For this review, take the finished solid that the model builds, in its own axes (mm). A direction names the side the tool comes from. Give positions to 0.01 mm unless a question says otherwise; leave off trailing zeros. Loops run counter-clockwise (first coordinate to the right, second up) from the corner with the lowest first, then second, coordinate; pieces in that order, holes last. Notation, with made-up numbers: (-27.5, 35.25) - (-22.5, 35.25) arc R36 ccw to (-22.5, 69.25) - close; hole circle Ø7 at (-38.5, 59.25). An arc over 180 degrees is marked (long way). Put each result on its own line as item: value. Start each with the question number.
from build123d import *

# Parameters (mm, degrees)
SKETCH1_W               = 58.6
SKETCH1_H               = 6.25
BOSS_EXTRUDE1_DEPTH     = 30
CUT_EXTRUDE1_DEPTH      = 67.128832592
CUT_EXTRUDE1_DEPTH_BACK = 35
SKETCH4_R               = 2.5
SKETCH4_W               = 15.6
SKETCH4_H               = 10.5
CUT_EXTRUDE2_DEPTH      = 4
CUT_EXTRUDE3_DEPTH      = 9.5
SKETCH6_W               = 15.6
SKETCH6_H               = 1
SKETCH6_H_2             = 0.5
CUT_EXTRUDE4_DEPTH      = 4
FILLET1_R               = 3
SKETCH7_R               = 1.65
CUT_EXTRUDE5_DEPTH      = 3


with BuildPart() as part:
    # Sketch1 → Boss-Extrude1 (new body)
    with BuildSketch(Plane(origin=(0, 0, 0), x_dir=(0, 0, -1), z_dir=(1, 0, 0))):
        with Locations((29.3, 3.125)):
            Rectangle(SKETCH1_W, SKETCH1_H)
    extrude(amount=BOSS_EXTRUDE1_DEPTH)

    # Sketch2 → Cut-Extrude1 (cut, two sides: drawn at the far end of the back side and taken through both)
    with BuildSketch(Plane.XY.offset(-CUT_EXTRUDE1_DEPTH_BACK)):
        with BuildLine():
            Line((5, 6.25), (25, 6.25))
            ThreePointArc((25, 6.25), (15, 2), (5, 6.25))
        make_face()
    extrude(amount=CUT_EXTRUDE1_DEPTH + CUT_EXTRUDE1_DEPTH_BACK, mode=Mode.SUBTRACT)

    # Sketch4 → Cut-Extrude2 (cut)
    with BuildSketch(Plane.XZ):
        with Locations(Location((15, -8.37, 0), (0, 0, 270))):
            Circle(SKETCH4_R)
        with Locations(Location((15, -15.02, 0), (0, 0, 270))):
            Circle(SKETCH4_R)
        with Locations(Location((15, -22.65, 0), (0, 0, 270))):
            Circle(SKETCH4_R)
        with Locations((15, -43.35)):
            Rectangle(SKETCH4_W, SKETCH4_H)
    extrude(amount=-CUT_EXTRUDE2_DEPTH, mode=Mode.SUBTRACT)

    # Sketch5 → Cut-Extrude3 (cut)
    with BuildSketch(Plane(origin=(0, 0, -58.6), x_dir=(-1, 0, 0), z_dir=(0, 0, -1))):
        Polygon((-9.85, 0.95), (-20.15, 0.95), (-17.975, 3.125), (-20.15, 5.3), (-9.85, 5.3), align=None)
    extrude(amount=-CUT_EXTRUDE3_DEPTH, mode=Mode.SUBTRACT)

    # Sketch6 → Cut-Extrude4 (cut)
    with BuildSketch(Plane.XZ):
        with Locations((15, -37.6)):
            Rectangle(SKETCH6_W, SKETCH6_H)
        with Locations((15, -48.85)):
            Rectangle(SKETCH6_W, SKETCH6_H_2)
    extrude(amount=-CUT_EXTRUDE4_DEPTH, mode=Mode.SUBTRACT)

    # Fillet1
    fillet1_edges = [part.edges().sort_by_distance(p)[0] for p in [
        (30, 3.125, -58.6),
        (30, 3.125, 0),
        (0, 3.125, -58.6),
        (0, 3.125, 0),
    ]]
    fillet(fillet1_edges, radius=FILLET1_R)

    # Sketch7 → Cut-Extrude5 (cut)
    with BuildSketch(Plane.XZ):
        with Locations(Location((3, -55.6, 0), (0, 0, 270))):
            Circle(SKETCH7_R)
        with Locations(Location((27, -55.6, 0), (0, 0, 90))):
            Circle(SKETCH7_R)
        with Locations(Location((27, -3, 0), (0, 0, 270))):
            Circle(SKETCH7_R)
        with Locations(Location((3, -3, 0), (0, 0, 90))):
            Circle(SKETCH7_R)
    extrude(amount=-CUT_EXTRUDE5_DEPTH, mode=Mode.SUBTRACT)


solid = part.part
1) Machinability: for faces 1 (the flat face through (0, 3, -29)), 2 (the flat face through (15, 2, -37.1)), 3 (the flat face through (15, 5, -35)), which of the approach directions +Z, -Z, +X, -X, +Y, -Y give a long, thin tool a straight path to every point of the face, cutting with its end or side? Answer none if there is none.
2) Take a section at B-B on z = -30.5. State the section outline as (x, y) points, and give its area (3 significant figures).
3) Wall thickness on probe 1 along Z at (x, y) = (15, 0.65); probe 2 along Z at (x, y) = (18, 0.75); probe 3 along X at (y, z) = (0.85, -15.02): over which ranges is each line inside the solid? List them lowest first.
4) Take a section at C-C on x = 8.75. State the section outline as (y, z) points, and give its area (3 significant figures).
5) Take a section at A-A on z = -22.65. State the section outline as (x, y) points, and give its area (3 significant figures).
6) Mouldability with a two-part tool opening along Y and no side actions: class faces 4 (the cylindrical face through (3.07, 1.48, -53.95)), 5 (the flat face through (27, 3, -56)), 6 (the flat face through (19.05, 4.2, -53.92)), 7 (the flat face through (15, 5.3, -54)) as released by +Y, released by -Y, zero draft, split by the parting line, or undercut.
7) Insertion check: P1, Ø2.5, axis at x = 3, z = -55.6, coming from the -Y side; P2, Ø8, axis at x = 15, z = -22.65, coming from the +Y side; P3, Ø3, axis at x = 15, z = -15.02, coming from the +Y side; P4, Ø6, axis at x = 19, z = -10, coming from the +Y side. Each pin has a flat end and moves straight along its axis. Give the tip position at first contact, or say it passes through.
Answers follow:
1. face 1: +Z, -Z, -X, +Y, -Y
1. face 2: -Y
1. face 3: +Z, +Y
2. outline: (0, 0) - (30, 0) - (30, 6.25) - (25, 6.25) arc R13.89 cw to (5, 6.25) - (0, 6.25) - close
2. area: 129 mm2
3. probe 1: -58.6 to -49.1, -37.1 to -25.15, -20.15 to -17.52, -12.52 to -10.87, -5.87 to 0
3. probe 2: -58.6 to -49.1, -37.1 to 0
3. probe 3: 0 to 12.5, 17.5 to 30
4. outline: (0, -58.6) - (6.25, -58.6) - (6.25, -35) - (3.49, -35) - (3.49, 0) - (0, 0) - (0, -37.1) - (4, -37.1) - (4, -49.1) - (0, -49.1) - close
4. area: 221 mm2
5. outline: (0, 0) - (12.5, 0) - (12.5, 2.23) arc R13.89 cw to (5, 6.25) - (0, 6.25) - close; (17.5, 0) - (30, 0) - (30, 6.25) - (25, 6.25) arc R13.89 cw to (17.5, 2.23) - close
5. area: 118 mm2
6. face 4: zero draft
6. face 5: released by -Y
6. face 6: undercut
6. face 7: undercut
7. P1: y = 3
7. P2: y = 2.59
7. P3: through
7. P4: y = 3.89
